```python
from build123d import *

# Parameters (mm, degrees)
SKETCH1_R                  = 6.4
BOSS_EXTRUDE1_DEPTH        = 100
F_10_24_TAPPED_HOLE1_D     = 3.7973
F_10_24_TAPPED_HOLE1_DEPTH = 12.83
F_10_24_TAPPED_HOLE1_TIP   = 1.140824014
F_10_24_TAPPED_HOLE2_D     = 3.7973
F_10_24_TAPPED_HOLE2_DEPTH = 12.83
F_10_24_TAPPED_HOLE2_TIP   = 1.140824014


with BuildPart() as part:
    # Sketch1 → Boss-Extrude1 (new body)
    with BuildSketch(Plane.XY):
        Circle(SKETCH1_R)
    extrude(amount=BOSS_EXTRUDE1_DEPTH)

    # #10-24 Tapped Hole1
    with Locations(Plane(origin=(0, 0, 0), x_dir=(-1, 0, 0), z_dir=(0, 0, -1))):
        with Locations((0, 0)):
            Hole(F_10_24_TAPPED_HOLE1_D / 2, depth=F_10_24_TAPPED_HOLE1_DEPTH)
            with Locations((0, 0, -(F_10_24_TAPPED_HOLE1_DEPTH + F_10_24_TAPPED_HOLE1_TIP / 2))):  # 118° drill point
                Cone(0, F_10_24_TAPPED_HOLE1_D / 2, F_10_24_TAPPED_HOLE1_TIP, mode=Mode.SUBTRACT)

    # #10-24 Tapped Hole2
    with Locations(Plane.XY.offset(100)):
        with Locations((0, 0)):
            Hole(F_10_24_TAPPED_HOLE2_D / 2, depth=F_10_24_TAPPED_HOLE2_DEPTH)
            with Locations((0, 0, -(F_10_24_TAPPED_HOLE2_DEPTH + F_10_24_TAPPED_HOLE2_TIP / 2))):  # 118° drill point
                Cone(0, F_10_24_TAPPED_HOLE2_D / 2, F_10_24_TAPPED_HOLE2_TIP, mode=Mode.SUBTRACT)


solid = part.part
```
Part model, mm, in its own coordinate system. A direction names the side the tool comes from. Give positions to 0.01 mm unless a question says otherwise; leave off trailing zeros. Loops run counter-clockwise (first coordinate to the right, second up) from the corner with the lowest first, then second, coordinate; pieces in that order, holes last. Notation, with made-up numbers: M 2.5,56 L 39.5,56 A16 ccw 39.5,75 Z; hole C -30,66 d8. An arc over 180 degrees is marked long. Return JSON: item names as keys, results as strings.
1) Saw through at A-A, the plane z = 78. List the corners of the cut face in (x, y).
Calculated:
{"outline": "C 0,0 d12.8"}
2) Saw through at B-B, the plane x = 4. List the corners of the cut face in (y, z), then the cut area to 3 significant figures.
Calculated:
{"outline": "M -5,0 L 5,0 L 5,100 L -5,100 Z", "area": "999 mm2"}
3) Saw through at C-C, the plane x = -3. List the corners of the cut face in (y, z), then the cut area to 3 significant figures.
Calculated:
{"outline": "M -5.65,0 L 5.65,0 L 5.65,100 L -5.65,100 Z", "area": "1,130 mm2"}
4) Flat gauge pins, fed straight in: pin 1 Ø1.5 at (y, z) = (2.5, 77) entering from -X; pin 2 Ø2 at (x, y) = (1, -1.5) entering from -Z; pin 3 Ø1.5 at (x, z) = (-5, 28) entering from -Y; pin 4 Ø2.5 at (x, y) = (0, 0) entering from -Z. Where does each tip first touch, or does it go through?
Calculated:
{"pin 1": "stops at x = -6.16", "pin 2": "stops at z = 0", "pin 3": "stops at y = -4.79", "pin 4": "stops at z = 13.22"}
5) Pull direction X, two halves, no side cores. Call faces 1 (the face through (-0.18, 0.28, 13.77)), 2 (the face through (-5.08, -3.89, 49.3)), 3 (the face through (1, 2, 0)): released by +X, released by -X, zero draft, split by the parting line, or undercut.
Calculated:
{"face 1": "undercut", "face 2": "split by the parting line", "face 3": "zero draft"}
6) 3-axis set-ups, long thin cutter, end or side, ignore diameter. For faces 4 (the face through (-1.8, 0.6, 93.5)), 5 (the face through (1.8, 0.6, 6.5)), 6 (the face through (1, 2, 100)): which of +Z, -Z, +X, -X, +Y, -Y reach the whole face in a straight line?
Calculated:
{"face 4": "+Z", "face 5": "-Z", "face 6": "+Z, +X, -X, +Y, -Y"}
7) Drill centre lines: line 1 (Y direction, x = 0, z = 97); line 2 (Y direction, x = 0.5, z = 78); line 3 (Y direction, x = -1.5, z = 4.5). Where is each one in solid material? Low to high.
Calculated:
{"line 1": "y = -6.4 to -1.9, 1.9 to 6.4", "line 2": "y = -6.38 to 6.38", "line 3": "y = -6.22 to -1.16, 1.16 to 6.22"}
